Design review of the part shown in the three views and the two pictorial views. Dimensions are in mm from the part's minimum x, y and z. Coordinates: 2 decimals unless noted, no trailing zeros. Loops run counter-clockwise (first coordinate to the right, second up) from the corner with the lowest first, then second, coordinate; pieces in that order, holes last.
Q1. For P1, Ø10, axis at x = 17.5, y = 29, coming from the -Z side, flat-tipped, find the tip position at first contact; note if it passes through.
Q2. Add section C-C on y = 99. Give the boundary of the cut face in (x, z).
Q3. Add section A-A on x = 28. Give the boundary of the cut face in (y, z).
Q4. Add section B-B on z = 2.9. Give the boundary of the cut face in (x, y), and give its area (3 significant figures).
Q5. Wall thickness on probe 1 along Y at (x, z) = (28, 2.3); probe 2 along Y at (x, z) = (31, 3.5) (1 decimal); probe 3 along X at (y, z) = (42.5, 2.55): over which ranges is each line inside the solid? List them lowest first.
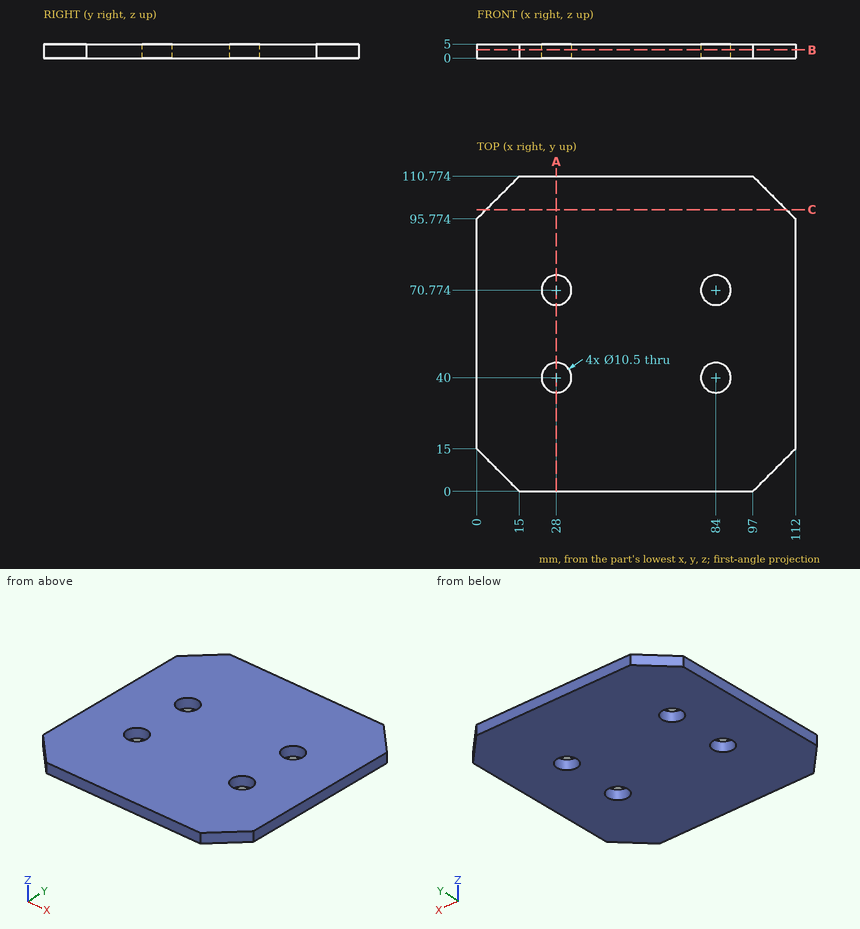
Entries:
1. P1: stops at z = 0
2. outline: (3.23, 0) - (108.77, 0) - (108.77, 5) - (3.23, 5) - close
3. outline: (0, 0) - (34.75, 0) - (34.75, 5) - (0, 5) - close; (45.25, 0) - (65.52, 0) - (65.52, 5) - (45.25, 5) - close; (76.02, 0) - (110.77, 0) - (110.77, 5) - (76.02, 5) - close
4. outline: (0, 15) - (15, 0) - (97, 0) - (112, 15) - (112, 95.77) - (97, 110.77) - (15, 110.77) - (0, 95.77) - close; hole circle Ø10.5 at (28, 40); hole circle Ø10.5 at (28, 70.77); hole circle Ø10.5 at (84, 40); hole circle Ø10.5 at (84, 70.77)
4. area: 11,600 mm2
5. probe 1: y = 0 to 34.75, 45.25 to 65.52, 76.02 to 110.77
5. probe 2: y = 0 to 35.7, 44.3 to 66.5, 75.1 to 110.8
5. probe 3: x = 0 to 23.38, 32.62 to 79.38, 88.62 to 112
